Could you check a few things on this model? Use its own coordinates, in mm. A direction names the side the tool comes from. Give positions to 0.01 mm unless a question says otherwise; leave off trailing zeros. Loops run counter-clockwise (first coordinate to the right, second up) from the corner with the lowest first, then second, coordinate; pieces in that order, holes last. Notation, with made-up numbers: (22.25, 53.5) - (66.25, 53.5) arc R31 ccw to (66.25, 77.5) - close; hole circle Ø10 at (21, -23). An arc over 180 degrees is marked (long way). One line per item, written item: value. Start each with the question number.
Q1. I want a section at C-C (x = 4.75). Please give me the cut outline in (y, z).
Q2. I want a section at A-A (y = 0). Please give me the cut outline in (x, z), then the cut area to 3 significant figures.
Q3. For faces 4 (the face through (0, 6, 0)), 5 (the face through (29, 0, 0)), which set-ups out of +Z, -Z, +X, -X, +Y, -Y let a thin tool reach every point of the face, with its end or its side?
Q4. If I drill on line 1 (Z direction, x = 7.75, y = 2.5); line 2 (Y direction, x = 29.6, z = 0); line 3 (Y direction, x = 4.25, z = -2.5), over which ranges is the centre line in solid material (lowest first)? Write a range as from..to.
Q5. If we mould it in two halves opening along Z, with no side actions, what happens to faces 1 (the face through (30, 0, 1)), 2 (the face through (29.49, -0.49, -0.63)), 3 (the face through (21.73, -2.92, -0.65))? For each: released by +Z, released by -Z, zero draft, split by the parting line, or undercut.
Q6. I want a section at D-D (x = 23). Please give me the cut outline in (y, z), then the cut area to 3 significant figures.
Q7. I'm going to push flat-ended pins straight in: P1, Ø1.5, axis at x = 23, y = 5, coming from the -Z side; P2, Ø1, axis at x = 3, y = -2, coming from the +Z side; P3, Ø5, axis at x = 16.5, z = 0.5, coming from the -Y side; P4, Ø3, axis at y = -6, z = -2.5, coming from the +X side. Where does each tip first touch, or does it pass through?
```python
from build123d import *


with BuildPart() as part:
    # Sketch 1 → Revolve 1 (revolve)
    with BuildSketch(Plane.XY, mode=Mode.PRIVATE) as revolve_1_sk:
        with BuildLine():
            Line((0, 0), (0, 7))
            ThreePointArc((0, 7), (0.292893219, 7.707106781), (1, 8))
            Line((1, 8), (2.978790918, 8))
            ThreePointArc((2.978790918, 8), (3.587095479, 7.937680303), (4.170127137, 7.753310373))
            Line((4.170127137, 7.753310373), (14, 3.5))
            Line((14, 3.5), (29.252387315, 2.499062082))
            ThreePointArc((29.252387315, 2.499062082), (29.783913457, 2.247629333), (30, 1.700779194))
            Line((30, 1.700779194), (30, 0.8))
            Line((30, 0.8), (29, 0.8))
            Line((29, 0.8), (29, 0))
            Line((29, 0), (0, 0))
        make_face()
    revolve(revolve_1_sk.sketch.rotate(Axis((30, 0, 0), (-1, 0, 0)), 270), axis=Axis((30, 0, 0), (-1, 0, 0)))

    # Sketch 2 → Cut-Revolve 1 (revolve, cut)
    with BuildSketch(Plane.XY):
        with BuildLine():
            Line((8.9865, 0), (-3.5865, 0))
            ThreePointArc((-3.5865, 0), (2.7, 6.2865), (8.9865, 0))
        make_face()
    revolve(axis=Axis((50, 0, 0), (-1, 0, 0)), mode=Mode.SUBTRACT)


solid = part.part
```
Worked answers:
1. outline: circle Ø15 at (0, 0); hole circle Ø11.89 at (0, 0)
2. outline: (0, -7) arc R1 ccw to (1, -8) - (2.98, -8) arc R3 ccw to (4.17, -7.75) - (14, -3.5) - (29.25, -2.5) arc R0.8 ccw to (30, -1.7) - (30, -0.8) - (29, -0.8) - (29, 0.8) - (30, 0.8) - (30, 1.7) arc R0.8 ccw to (29.25, 2.5) - (14, 3.5) - (4.17, 7.75) arc R3 ccw to (2.98, 8) - (1, 8) arc R1 ccw to (0, 7) - (0, 5.68) arc R6.29 cw (long way) to (0, -5.68) - close
2. area: 175 mm²
3. face 4: +Z, -Z, -X, +Y, -Y
3. face 5: +X
4. line 1: z = -5.68..-2.79, 2.79..5.68
4. line 2: y = -2.39..-0.8, 0.8..2.39
4. line 3: y = -7.3..-5.56, 5.56..7.3
5. face 1: zero draft
5. face 2: undercut
5. face 3: split by the parting line
6. outline: circle Ø5.82 at (0, 0)
6. area: 26.6 mm²
7. P1: passes through
7. P2: stops at z = 7.86
7. P3: stops at y = -3.5
7. P4: stops at x = 10.53
